```python
from build123d import *

# Parameters (mm, degrees)
BOX001_W        = 47
BOX001_H        = 52
BOX001_DEPTH    = 3
SKETCH_R        = 1.75
SKETCH_W        = 26
SKETCH_H        = 24
POCKET004_DEPTH = 5
SKETCH001_W     = 66.159115
SKETCH001_H     = 64.322982
POCKET005_DEPTH = 5
FILLET014_R     = 4
BOX002_W        = 40.5
BOX002_H        = 3
BOX002_DEPTH    = 10.5
FILLET015_R     = 2
SKETCH002_R     = 1.75
POCKET006_DEPTH = 5


with BuildPart() as fillet_tongue_base:
    # Box001 → Box001 (new body)
    with BuildSketch(Plane(origin=(-23.5, 56, -34), x_dir=(1, 0, 0), z_dir=(0, 0, 1))):
        with Locations((23.5, 26)):
            Rectangle(BOX001_W, BOX001_H)
    extrude(amount=BOX001_DEPTH)

    # Sketch → Pocket004 (cut)
    with BuildSketch(Plane(origin=(-23.5, 56, -31), x_dir=(1, 0, 0), z_dir=(0, 0, 1))):
        with Locations((7.25, 36.025334)):
            Circle(SKETCH_R)
        with Locations((39.25, 36.025334)):
            Circle(SKETCH_R)
        with Locations((23.25, 36.775334)):
            Rectangle(SKETCH_W, SKETCH_H)
    extrude(amount=-POCKET004_DEPTH, mode=Mode.SUBTRACT)

    # Sketch001 → Pocket005 (cut)
    with BuildSketch(Plane(origin=(-23.5, 56, -31), x_dir=(1, 0, 0), z_dir=(0, 0, 1))):
        with Locations((23.771638, 27.147535)):
            Rectangle(SKETCH001_W, SKETCH001_H)
        with BuildLine():
            Line((0, 36), (9.237604, 52))
            Line((9.237604, 52), (37.762396, 52))
            Line((37.762396, 52), (47, 36))
            Line((47, 36), (38.847126, 21.878809))
            ThreePointArc((38.847126, 21.878809), (37.448559, 15.173629), (40.30581, 8.948554))
            ThreePointArc((43.75, 3), (42.36158, 6.167474), (40.30581, 8.948554))
            Line((43.75, 0), (43.75, 3))
            Line((3.25, 0), (43.75, 0))
            Line((3.25, 0), (3.25, 3))
            ThreePointArc((6.69419, 8.948554), (4.63842, 6.167474), (3.25, 3))
            ThreePointArc((6.69419, 8.948554), (9.551428, 15.17363), (8.152874, 21.878809))
            Line((0, 36), (8.152874, 21.878809))
        make_face(mode=Mode.SUBTRACT)
    extrude(amount=-POCKET005_DEPTH, mode=Mode.SUBTRACT)

    # Fillet014
    fillet014_edges = [fillet_tongue_base.edges().sort_by_distance(p)[0] for p in [
        (-14.262396, 108, -32.5),
        (-23.5, 92, -32.5),
        (14.262396, 108, -32.5),
        (23.5, 92, -32.5),
    ]]
    fillet(fillet014_edges, radius=FILLET014_R)


with BuildPart() as obj1:
    # Box002 → Box002 (new body)
    with BuildSketch(Plane(origin=(-20.25, 56, -31), x_dir=(1, 0, 0), z_dir=(0, 0, 1))):
        with Locations((20.25, 1.5)):
            Rectangle(BOX002_W, BOX002_H)
    extrude(amount=BOX002_DEPTH)

    # Fillet015
    fillet015_edges = [obj1.edges().sort_by_distance(p)[0] for p in [
        (-20.25, 57.5, -20.5),
        (20.25, 57.5, -20.5),
    ]]
    fillet(fillet015_edges, radius=FILLET015_R)

    # Sketch002 → Pocket006 (cut)
    with BuildSketch(Plane(origin=(0, 59, 0), x_dir=(-1, 0, 0), z_dir=(0, 1, 0))):
        with Locations((0, -25.6)):
            Circle(SKETCH002_R)
    extrude(amount=-POCKET006_DEPTH, mode=Mode.SUBTRACT)

    # Fusion005: union Fillet_tongue_base
    add(fillet_tongue_base.part)


solid = obj1.part
```
Here's how the part is built. I have some questions about the finished solid (model axes, mm). A direction names the side the tool comes from. Coordinates: 2 decimals unless noted, no trailing zeros. Write each loop counter-clockwise with the first axis right and the second up, starting at its lowest first coordinate (ties: lowest second). Pieces come first, ordered by that corner, then holes. Notation, with made-up numbers: M -36.75,50.5 L -28.75,50.5 A17 ccw -28.75,81.5 Z; hole C 32,24.5 d9. An arc over 180 degrees is marked long. Answer as CSV lines item,"result". Start each with the question number.
Q1. Suppose I cut it at C-C, the plane x = -5. List the corners of the cut face in (y, z) for me.
Q2. Suppose I cut it at D-D, the plane z = -32.75. List the corners of the cut face in (x, y) for me.
Q3. If we mould it in two halves opening along Z, with no side actions, what happens to faces 1 (the cylindrical face through (0.38, 57.52, -27.31)), 2 (the flat face through (0, 58, -20.5)), 3 (the flat face through (-18.895, 84.024, -32.479))? For each: pulls with the +Z half, pulls with the -Z half, needs draft (parallel to the pull), parting line crosses it, or undercut.
Q4. Suppose I cut it at B-B, the plane x = 0. List the corners of the cut face in (y, z) for me.
Q5. Suppose I cut it at A-A, the plane z = -25.6. List the corners of the cut face in (x, y) for me.
Q6. Will these pins go through, and if not, where does the flat tip stop? pin 1 Ø6 at (x, z) = (-12, -25) entering from +Y; pin 2 Ø1.5 at (x, y) = (2, 81) entering from +Z; pin 3 Ø2.5 at (y, z) = (57.5, -29.5) entering from -X.
Q7. I need wall thicknesses on probe 1 along Y at (x, z) = (-16.25, -31.65); probe 2 along Y at (x, z) = (-3, -32); probe 3 along Z at (x, y) = (0, 57.65). Which ranges of each line are inside material? Lowest first, please. Write a range as [from, to].
Q8. For faces 4 (the flat face through (0, 78, -31)), 5 (the flat face through (-20.25, 57, -28)), 6 (the cylindrical face through (18.9, 62.1, -32.5)), which set-ups out of +Z, -Z, +X, -X, +Y, -Y let a thin tool reach every point of the face, with its end or its side?
Entries:
1,outline,"M 56,-34 L 80.78,-34 L 80.78,-31 L 59,-31 L 59,-20.5 L 56,-20.5 Z; M 104.78,-34 L 108,-34 L 108,-31 L 104.78,-31 Z"
2,outline,"M -22.35,90 L -15.35,77.88 A10.95 cw -16.81,64.95 A15.51 ccw -20.25,59 L -20.25,56 L 20.25,56 L 20.25,59 A15.51 ccw 16.81,64.95 A10.95 cw 15.35,77.88 L 22.35,90 A4 ccw 22.35,94 L 15.42,106 A4 ccw 11.95,108 L -11.95,108 A4 ccw -15.42,106 L -22.35,94 A4 ccw Z; hole C -16.25,92.03 d3.5; hole M -13.25,80.78 L 12.75,80.78 L 12.75,104.78 L -13.25,104.78 Z; hole C 15.75,92.03 d3.5"
3,face 1,"undercut"
3,face 2,"pulls with the +Z half"
3,face 3,"needs draft"
4,outline,"M 56,-34 L 80.78,-34 L 80.78,-31 L 59,-31 L 59,-27.35 L 56,-27.35 Z; M 56,-23.85 L 59,-23.85 L 59,-20.5 L 56,-20.5 Z; M 104.78,-34 L 108,-34 L 108,-31 L 104.78,-31 Z"
5,outline,"M -20.25,56 L -1.75,56 L -1.75,59 L -20.25,59 Z; M 1.75,56 L 20.25,56 L 20.25,59 L 1.75,59 Z"
6,pin 1,"stops at y = 59"
6,pin 2,"stops at z = -31"
6,pin 3,"stops at x = -20.25"
7,probe 1,"y = [56, 65.6], [79.44, 90.28], [93.78, 104.56]"
7,probe 2,"y = [56, 80.78], [104.78, 108]"
7,probe 3,"z = [-34, -27.35], [-23.85, -20.5]"
8,face 4,"+Z, +X, -X, +Y"
8,face 5,"+Z, -Z, -X, -Y"
8,face 6,"+Z, -Z, +X"
